Could you check a few things on this drawing? It's one solid part, dimensions in mm from its lowest x, y, z. A direction names the side the tool comes from. Round coordinates to 2 decimals unless told otherwise and drop trailing zeros. Write each loop counter-clockwise with the first axis right and the second up, starting at its lowest first coordinate (ties: lowest second). Pieces come first, ordered by that corner, then holes. Notation, with made-up numbers: (54.25, 27) - (111.25, 27) arc R35 cw to (111.25, 63) - close; hole circle Ø11 at (78.25, 86.25). An arc over 180 degrees is marked (long way). Put each result on its own line as item: value.
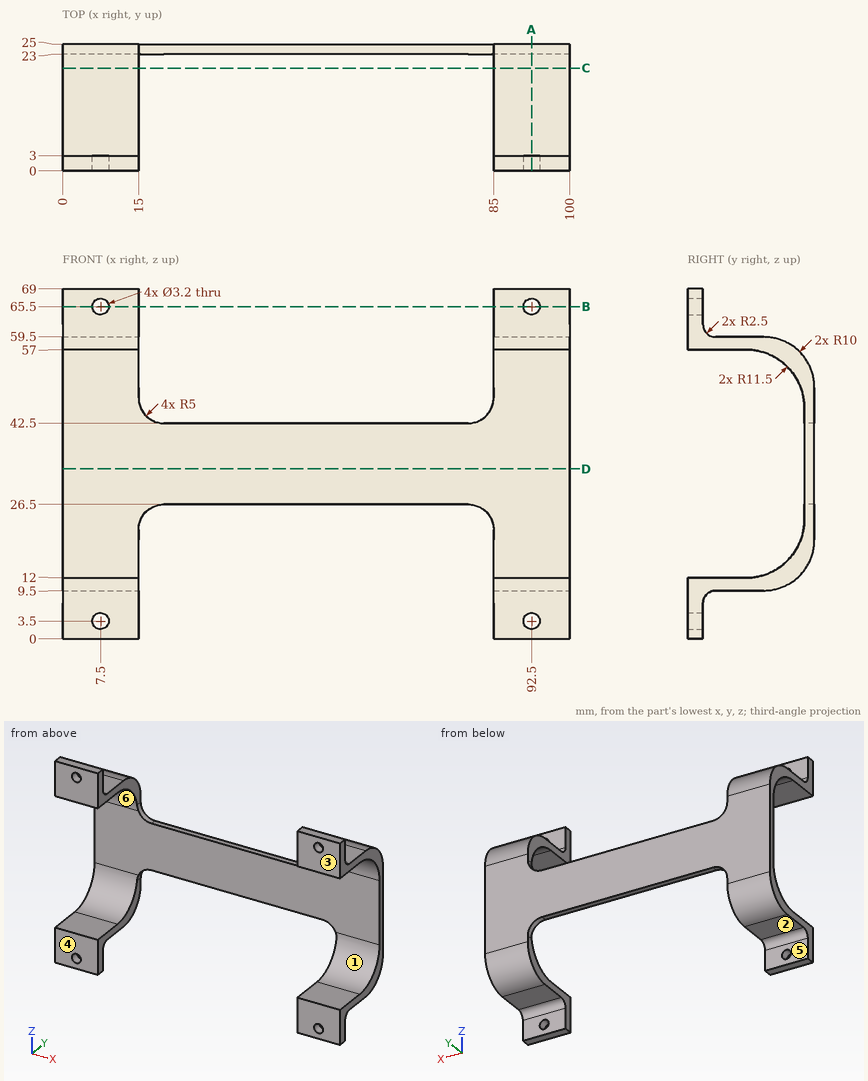
(1) If we mould it in two halves opening along Z, with no side actions, what happens to the marked faces 1, 2 and 3? For each: pulls with the +Z half, pulls with the -Z half, needs draft (parallel to the pull), parting line crosses it, or undercut.
Values found:
face 1: undercut
face 2: pulls with the -Z half
face 3: needs draft
(2) Imagine slicing it at C-C, the plane y = 20.25. List the corners of the cut face in (x, z) for me, then the cut area to 3 significant figures.
Values found:
outline: (0, 10.99) - (15, 10.99) - (15, 16.04) - (0, 16.04) - close; (0, 52.96) - (15, 52.96) - (15, 58.01) - (0, 58.01) - close; (85, 10.99) - (100, 10.99) - (100, 16.04) - (85, 16.04) - close; (85, 52.96) - (100, 52.96) - (100, 58.01) - (85, 58.01) - close
area: 303 mm^2
(3) Imagine slicing it at A-A, the plane x = 92.5. List the corners of the cut face in (y, z) for me.
Values found:
outline: (0, 0) - (3, 0) - (3, 1.9) - (0, 1.9) - close; (0, 5.1) - (3, 5.1) - (3, 7) arc R2.5 cw to (5.5, 9.5) - (15, 9.5) arc R10 ccw to (25, 19.5) - (25, 49.5) arc R10 ccw to (15, 59.5) - (5.5, 59.5) arc R2.5 cw to (3, 62) - (3, 63.9) - (0, 63.9) - (0, 57) - (11.5, 57) arc R11.5 cw to (23, 45.5) - (23, 23.5) arc R11.5 cw to (11.5, 12) - (0, 12) - close; (0, 67.1) - (3, 67.1) - (3, 69) - (0, 69) - close
(4) I'm going to push flat-ended pins straight in: pin 1 (7.5 mm diameter, centred on x = 94, z = 3.5, fed in from +Y); pin 2 (1.6 mm diameter, centred on x = 56, y = 24, fed in from -Z); pin 3 (12 mm diameter, centred on x = 18.5, z = 28.5, fed in from -Y). Where does each tip first touch, or does it pass through?
Values found:
pin 1: stops at y = 3.01
pin 2: stops at z = 26.5
pin 3: stops at y = 23
(5) For the marked faces 4, 5 and 6, which set-ups out of +Z, -Z, +X, -X, +Y, -Y let a thin tool reach every point of the face, with its end or its side?
Values found:
face 4: +Z, -Z, +X, -X, -Y
face 5: -Z, +X, -X, +Y
face 6: +X, -X, -Y
(6) Please list where these lines run through material, in increasing order: probe 1 along Z at (x, y) = (92.5, 1.5); probe 2 along X at (y, z) = (1.25, 65.5); probe 3 along Y at (x, z) = (93, 40). Write a range as from..to.
Values found:
probe 1: z = 0..1.9, 5.1..12, 57..63.9, 67.1..69
probe 2: x = 0..5.9, 9.1..15, 85..90.9, 94.1..100
probe 3: y = 23..25
(7) Imagine slicing it at D-D, the plane z = 33.5. List the corners of the cut face in (x, y) for me, then the cut area to 3 significant figures.
Values found:
outline: (0, 23) - (100, 23) - (100, 25) - (0, 25) - close
area: 200 mm^2
(8) Imagine slicing it at B-B, the plane z = 65.5. List the corners of the cut face in (x, y) for me, then the cut area to 3 significant figures.
Values found:
outline: (0, 0) - (5.9, 0) - (5.9, 3) - (0, 3) - close; (9.1, 0) - (15, 0) - (15, 3) - (9.1, 3) - close; (85, 0) - (90.9, 0) - (90.9, 3) - (85, 3) - close; (94.1, 0) - (100, 0) - (100, 3) - (94.1, 3) - close
area: 70.8 mm^2
